Verification items for the finished model (mm, model axes). A direction names the side the tool comes from. Coordinates: 2 decimals unless noted, no trailing zeros. Write each loop counter-clockwise with the first axis right and the second up, starting at its lowest first coordinate (ties: lowest second). Pieces come first, ordered by that corner, then holes. Notation, with made-up numbers: (41, -27) -> (50, -27) arc R12 cw to (50, -6) -> close; hole circle Ø10 at (18, 67.25). An arc over 180 degrees is marked (long way). Answer in a Markdown table with one row per item.
```python
from build123d import *

# Parameters (mm, degrees)
SKETCH1_R                = 8.3
SKETCH1_R_2              = 6.3
BOSS_EXTRUDE1_DEPTH      = 95
SKETCH3_R                = 8.3
BOSS_EXTRUDE2_DEPTH      = 3
SKETCH5_W                = 16.6
SKETCH5_H                = 16.6
BOSS_EXTRUDE4_DEPTH      = 7
CUT_EXTRUDE1_DEPTH       = 107.627623063
FILLET1_R                = 4.1
SKETCH4_R                = 6.3
SKETCH4_R_2              = 1.5
CUT_EXTRUDE3_DEPTH       = 3
BOSS_EXTRUDE6_START      = 2
SKETCH8_R                = 1.5
BOSS_EXTRUDE6_DEPTH      = 2
BOSS_EXTRUDE7_START      = -0.774045
BOSS_EXTRUDE7_DEPTH      = 7.774045
F_3_0_3_DIAMETER_HOLE1_D = 3
F_3_0_3_DIAMETER_HOLE2_D = 3
F_3_0_3_DIAMETER_HOLE3_D = 3
CUT_EXTRUDE4_START       = -105
CUT_EXTRUDE4_DEPTH       = 105


# Read off the part's stored shape, not the designer's step: Cut-Extrude4
with BuildPart() as part:
    # Sketch1 → Boss-Extrude1 (new body)
    with BuildSketch(Plane(origin=(0, 0, 0), x_dir=(1, 0, 0), z_dir=(0, 1, 0))):
        with Locations(Location((0, 0, 0), (0, 0, 270))):
            Circle(SKETCH1_R)
        with Locations(Location((0, 0, 0), (0, 0, 270))):
            Circle(SKETCH1_R_2, mode=Mode.SUBTRACT)
    extrude(amount=BOSS_EXTRUDE1_DEPTH)

    # Sketch3 → Boss-Extrude2 (add)
    with BuildSketch(Plane(origin=(0, 95, 0), x_dir=(1, 0, 0), z_dir=(0, 1, 0))):
        with Locations(Location((0, 0, 0), (0, 0, 270))):
            Circle(SKETCH3_R)
    extrude(amount=BOSS_EXTRUDE2_DEPTH)

    # Sketch5 → Boss-Extrude4 (add)
    with BuildSketch(Plane(origin=(0, 98, 0), x_dir=(1, 0, 0), z_dir=(0, 1, 0))):
        Rectangle(SKETCH5_W, SKETCH5_H)
    extrude(amount=BOSS_EXTRUDE4_DEPTH)

    # Sketch6 → Cut-Extrude1 (cut, through all)
    with BuildSketch(Plane.XY.offset(8.3)):
        Polygon((4.1, 10), (0, 10), (-4.1, 10), (-4.1, 88), (4.1, 88), align=None)
    extrude(amount=-CUT_EXTRUDE1_DEPTH, mode=Mode.SUBTRACT)

    # Fillet1
    fillet1_edges = [part.edges().sort_by_distance(p)[0] for p in [
        (4.1, 88, 5.999975859),
        (4.1, 88, -5.999975859),
        (-4.1, 88, 5.999975859),
        (-4.1, 88, -5.999975859),
        (4.1, 10, -5.999975859),
        (4.1, 10, 5.999975859),
        (-4.1, 10, -5.999975859),
        (-4.1, 10, 5.999975859),
    ]]
    fillet(fillet1_edges, radius=FILLET1_R - 0.0001)  # a hair under: the kernel refuses the full size

    # Sketch4 → Cut-Extrude3 (cut)
    with BuildSketch(Plane(origin=(0, 95, 0), x_dir=(-1, 0, 0), z_dir=(0, -1, 0))):
        with Locations(Location((0, 0, 0), (0, 0, 90))):
            Circle(SKETCH4_R)
        with Locations(Location((0, 0, 0), (0, 0, 90))):
            Circle(SKETCH4_R_2, mode=Mode.SUBTRACT)
    extrude(amount=-CUT_EXTRUDE3_DEPTH, mode=Mode.SUBTRACT)

    # Sketch8 → Boss-Extrude6 (add)
    with BuildSketch(Plane(origin=(0, 95, 0), x_dir=(-1, 0, 0), z_dir=(0, -1, 0)).offset(BOSS_EXTRUDE6_START)):
        with Locations(Location((0, 0, 0), (0, 0, 90))):
            Circle(SKETCH8_R)
    extrude(amount=-BOSS_EXTRUDE6_DEPTH)

    # Sketch9 → Boss-Extrude7 (add)
    with BuildSketch(Plane.ZY.offset(8.3).offset(BOSS_EXTRUDE7_START)):
        Polygon((0, 0), (3.5, 0), (3.5, 105), (-3.5, 105), (-3.5, 0), align=None)
    boss_extrude7 = extrude(amount=BOSS_EXTRUDE7_DEPTH)

    # Mirror1: Boss-Extrude7 across plane
    add(boss_extrude7.mirror(Plane(origin=(0, 0, 0), x_dir=(0, 0, 1), z_dir=(1, 0, 0))))

    # Ø3.0 (3) Diameter Hole1 (through all)
    with Locations(Plane.XY.offset(8.3)):
        with Locations((0, 101.5)):
            Hole(F_3_0_3_DIAMETER_HOLE1_D / 2)

    # Ø3.0 (3) Diameter Hole2 (through all)
    with Locations(Plane.XY.offset(3.5)):
        with Locations((11.8, 85), (11.8, 11)):
            f_3_0_3_diameter_hole2 = Hole(F_3_0_3_DIAMETER_HOLE2_D / 2)

    # Ø3.0 (3) Diameter Hole3 (through all)
    with Locations(Plane(origin=(0, 0, -3.5), x_dir=(-1, 0, 0), z_dir=(0, 0, -1))):
        with Locations((-11.8, 65), (-11.8, 51)):
            Hole(F_3_0_3_DIAMETER_HOLE3_D / 2)

    # Mirror2: Ø3.0 (3) Diameter Hole2 across plane
    add(f_3_0_3_diameter_hole2.mirror(Plane(origin=(0, 0, 0), x_dir=(0, 0, 1), z_dir=(1, 0, 0))), mode=Mode.SUBTRACT)

    # Cut-Extrude4 outline → Cut-Extrude4 (cut)
    with BuildSketch(Plane(origin=(0, 0, 0), x_dir=(-1, 0, 0), z_dir=(0, -1, 0)).offset(CUT_EXTRUDE4_START)):
        with BuildLine():
            ThreePointArc((-4, 0), (0, -4), (4, 0))
            Line((4, 0), (15.3, 0))
            Line((15.3, 0), (15.3, 3.5))
            Line((15.3, 3.5), (8.3, 3.5))
            Line((8.3, 3.5), (8.3, 8.3))
            Line((8.3, 8.3), (-8.3, 8.3))
            Line((-8.3, 8.3), (-8.3, 3.5))
            Line((-8.3, 3.5), (-15.3, 3.5))
            Line((-15.3, 3.5), (-15.3, 0))
            Line((-15.3, 0), (-4, 0))
        make_face()
    extrude(amount=CUT_EXTRUDE4_DEPTH, mode=Mode.SUBTRACT)


solid = part.part
```
1. Section check A-A, the plane z = 1.5. Record the boundary of the cut face in (x, y).
Geometry says:
| item | result |
|---|---|
| outline | (-15.3, 0) -> (-6.12, 0) -> (-6.12, 98) -> (-3.71, 98) -> (-3.71, 105) -> (-15.3, 105) -> close; (3.71, 98) -> (6.12, 98) -> (6.12, 0) -> (15.3, 0) -> (15.3, 105) -> (3.71, 105) -> close; hole circle Ø3 at (-11.8, 11); hole circle Ø3 at (-11.8, 85); hole circle Ø3 at (11.8, 11); hole circle Ø3 at (11.8, 51); hole circle Ø3 at (11.8, 65); hole circle Ø3 at (11.8, 85) |
2. Thickness scan on line 1 (Y direction, x = -11.8, z = 1.75); line 2 (X direction, y = 101.5, z = 6.2); line 3 (Y direction, x = 11.8, z = 2.55). Record the ranges inside material, lowest first. Write a range as from..to.
Geometry says:
| item | result |
|---|---|
| line 1 | 0..9.5, 12.5..83.5, 86.5..105 |
| line 2 | -8.3..-1.5, 1.5..8.3 |
| line 3 | 0..9.5, 12.5..49.5, 52.5..63.5, 66.5..83.5, 86.5..105 |
3. Tool access check on faces 5 (the flat face through (0, 98, 5)), 6 (the flat face through (4.1, 49, 6)), 7 (the flat face through (-6, 98, 6)). Record the directions out of +Z, -Z, +X, -X, +Y, -Y that give a thin tool (end or side, any length) a straight path to the whole face; none if there is none.
Geometry says:
| item | result |
|---|---|
| face 5 | -Z, -Y |
| face 6 | +Z, -Z |
| face 7 | +Z, -X, -Y |
4. Mould release check, pull along X, two halves, no side actions. Record for faces 1 (the flat face through (-15.3, 53, 2)), 2 (the cylindrical face through (-11.995, 86.487, 1.725)), 3 (the flat face through (11, 53, 0)), 4 (the cylindrical face through (13.3, 11.07, 1.73)): released by +X, released by -X, zero draft, split by the parting line, or undercut.
Geometry says:
| item | result |
|---|---|
| face 1 | released by -X |
| face 2 | undercut |
| face 3 | zero draft |
| face 4 | undercut |
5. Section check B-B, the plane y = 51. Record the boundary of the cut face in (x, z).
Geometry says:
| item | result |
|---|---|
| outline | (-15.3, 0) -> (-6.3, 0) arc R6.3 cw to (-4.1, 4.78) -> (-4.1, 7.22) arc R8.3 ccw to (-7.53, 3.5) -> (-15.3, 3.5) -> close; (4.1, 4.78) arc R6.3 cw to (6.3, 0) -> (10.3, 0) -> (10.3, 3.5) -> (7.53, 3.5) arc R8.3 ccw to (4.1, 7.22) -> close; (13.3, 0) -> (15.3, 0) -> (15.3, 3.5) -> (13.3, 3.5) -> close |
6. Depth check by flat-ended pin: P1, Ø4, axis at x = -13, y = 63.5, coming from the +Z side; P2, Ø1.4, axis at y = 100.5, z = 5.5, coming from the +X side; P3, Ø4, axis at x = -5.5, y = 42.5, coming from the +Z side; P4, Ø4, axis at x = 11.8, y = 11, coming from the -Z side. Enter the tip coordinate at first touch or a pass-through.
Geometry says:
| item | result |
|---|---|
| P1 | z = 3.5 |
| P2 | x = 8.3 |
| P3 | z = 7.22 |
| P4 | z = 0 |
7. Section check C-C, the plane y = 91. Record the boundary of the cut face in (x, z).
Geometry says:
| item | result |
|---|---|
| outline | (-15.3, 0) -> (-6.3, 0) arc R6.3 cw to (6.3, 0) -> (15.3, 0) -> (15.3, 3.5) -> (7.53, 3.5) arc R8.3 ccw to (-7.53, 3.5) -> (-15.3, 3.5) -> close |
